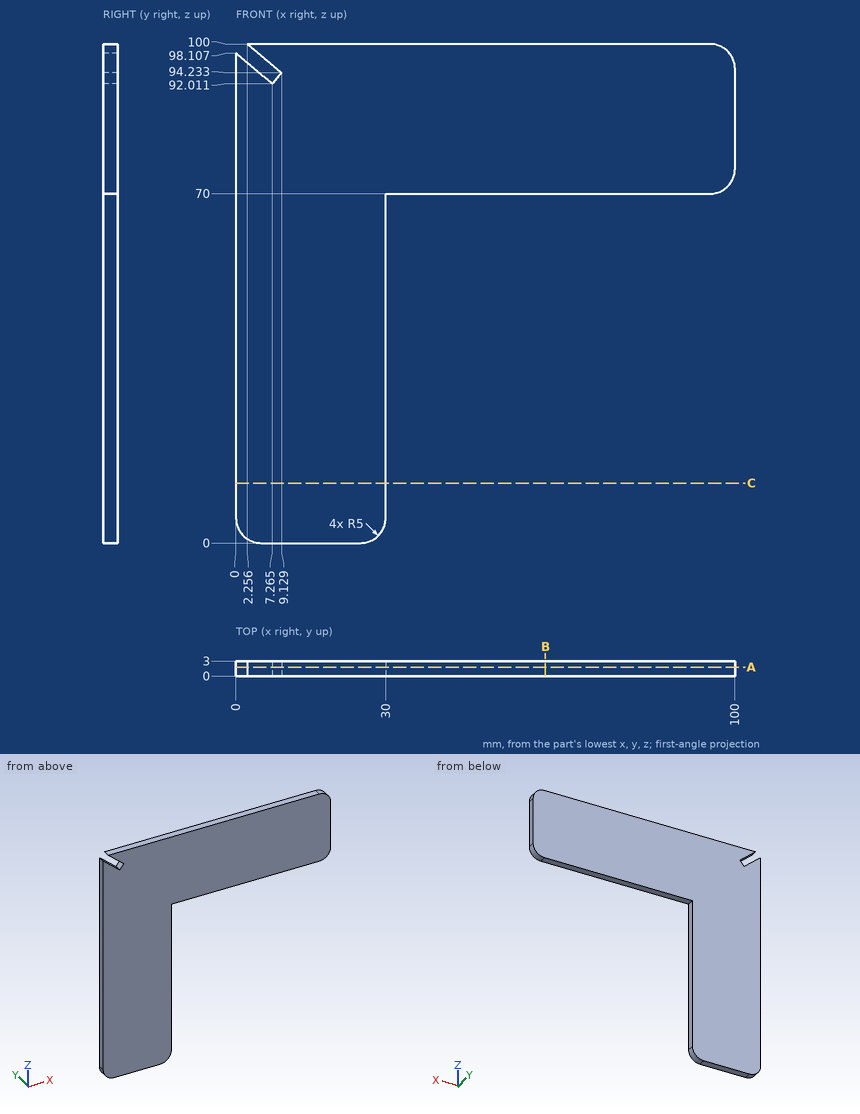
Study the drawing (mm; zero at the part's minimum x, y, z) and answer. Coordinates: 2 decimals unless noted, no trailing zeros. Loops run counter-clockwise (first coordinate to the right, second up) from the corner with the lowest first, then second, coordinate; pieces in that order, holes last. Notation, with made-up numbers: (75, 13.25) -> (94, 13.25) arc R32 ccw to (94, 47.25) -> close; hole circle Ø5 at (52.5, 79.5). An arc over 180 degrees is marked (long way). Write each question's results on one line, items separated by ' | '. Start each with the question number.
1) Find section B-B on x = 62. Determine the outline of the cut face in (y, z).
2) A flat-ended cylindrical pin translates along its axis: P1, Ø0.9, axis at y = 1, z = 32, coming from the +X side. Find the tip coordinate at first contact, or state that the pin passes through.
3) Consider line 1 along Z through (x, y) = (67.5, 1.25); line 2 along X through (y, z) = (1.4, 39); line 3 along Z through (x, y) = (8.5, 2.5) (1 decimal). Determine where each line is inside the solid, lowest interval first.
4) Find section C-C on z = 12. Determine the outline of the cut face in (x, y).
5) Find section A-A on y = 1.8. Determine the outline of the cut face in (x, z) (1 decimal).
Response values:
1) outline: (0, 70) -> (3, 70) -> (3, 100) -> (0, 100) -> close
2) P1: stops at x = 30
3) line 1: z = 70 to 100 | line 2: x = 0 to 30 | line 3: z = 0 to 93.5, 94.8 to 100
4) outline: (0, 0) -> (30, 0) -> (30, 3) -> (0, 3) -> close
5) outline: (0, 5) arc R5 ccw to (5, 0) -> (25, 0) arc R5 ccw to (30, 5) -> (30, 70) -> (95, 70) arc R5 ccw to (100, 75) -> (100, 95) arc R5 ccw to (95, 100) -> (2.3, 100) -> (9.1, 94.2) -> (7.3, 92) -> (0, 98.1) -> close
